Could you check a few things on this drawing? It's one solid part, dimensions in mm from its lowest x, y, z. A direction names the side the tool comes from. Give positions to 0.01 mm unless a question says otherwise; leave off trailing zeros. Write each loop counter-clockwise with the first axis right and the second up, starting at its lowest first coordinate (ties: lowest second). Pieces come first, ordered by that corner, then holes. Notation, with made-up numbers: M -6,-2 L 13,-2 A21 cw 13,7 Z; hole C 62.25,71.5 d3. An arc over 180 degrees is marked long. Use CSV: the item, a comma, the result in double quotes. Start each with the question number.
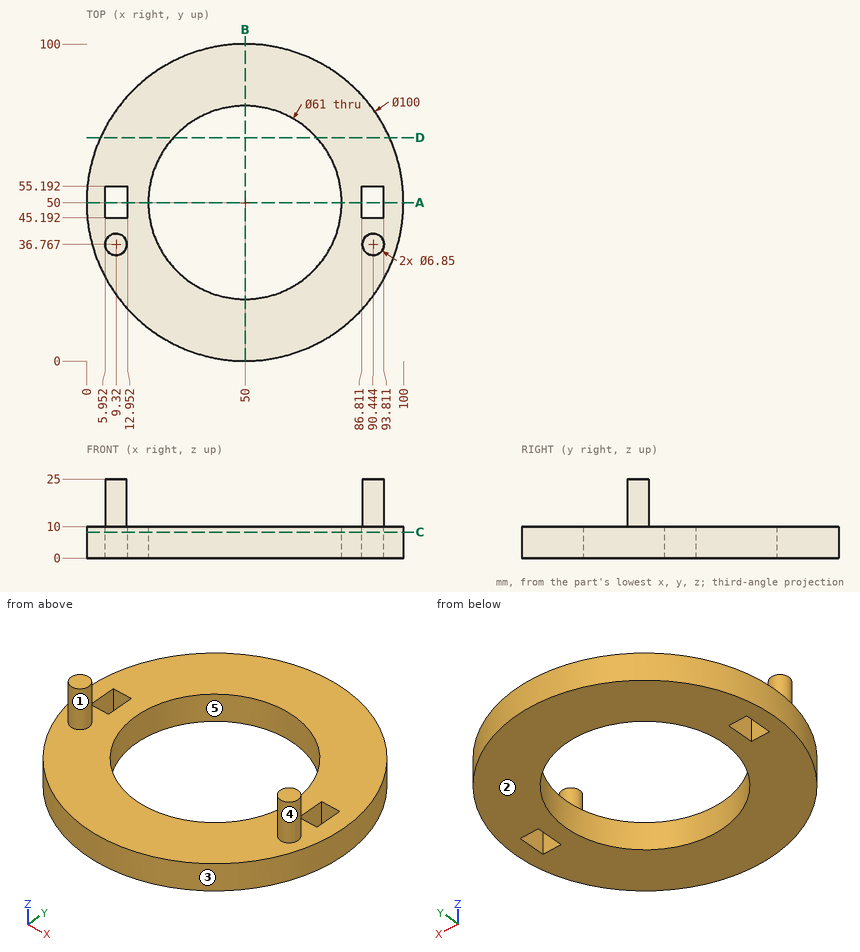
(1) Please list where these lines run through material, in increasing order: L1, parallel to Y at x = 50, z = 2.5; L2, parallel to Z at x = 10.5, y = 64; L3, parallel to Y at x = 88, z = 4.5 (1 decimal). Write a range as [from, to].
(2) I want a section at B-B (x = 50). Write out the boundary of the cut face in (y, z), and give its area (3 significant figures).
(3) Will these pins go through, and if not, where does the flat tip stop? pin 1 Ø10 at (y, z) = (13, 11.5) entering from -X (1 decimal); pin 2 Ø1 at (x, z) = (45.5, 8) entering from -Y; pin 3 Ø7.5 at (x, z) = (8, 4.5) entering from -Y; pin 4 Ø11 at (y, z) = (50.5, 3.5) entering from -X.
(4) Which directions (+Z, -Z, +X, -X, +Y, -Y) give clear straight access to the entire face, cutting with the end or side of a thin tool? Please do the marked faces 4 and 5.
(5) I want a section at C-C (z = 8.25). Write out the boundary of the cut face in (x, y), and give its area (3 significant figures).
(6) Thinking about a two-plate mould opening in X: for the marked faces 1, 2 and 3, which applies, released by +X, released by -X, zero draft, split by the parting line, or undercut?
(7) I want a section at D-D (y = 70.5). Write out the boundary of the cut face in (x, z) (1 decimal).
(8) I want a section at A-A (y = 50). Write out the boundary of the cut face in (x, z), and give its area (3 significant figures).
Geometry results:
1,L1,"y = [0, 19.5], [80.5, 100]"
1,L2,"z = [0, 10]"
1,L3,"y = [17.5, 45.2], [55.2, 82.5]"
2,outline,"M 0,0 L 19.5,0 L 19.5,10 L 0,10 Z; M 80.5,0 L 100,0 L 100,10 L 80.5,10 Z"
2,area,"390 mm2"
3,pin 1,"stops at x = 11.8"
3,pin 2,"stops at y = 0.16"
3,pin 3,"stops at y = 17.8"
3,pin 4,"stops at x = 0"
4,face 4,"+Z"
4,face 5,"+Z, -Z"
5,outline,"C 50,50 d100; hole M 5.95,45.19 L 12.95,45.19 L 12.95,55.19 L 5.95,55.19 Z; hole C 50,50 d61; hole M 86.81,45.19 L 93.81,45.19 L 93.81,55.19 L 86.81,55.19 Z"
5,area,"4,790 mm2"
6,face 1,"undercut"
6,face 2,"zero draft"
6,face 3,"split by the parting line"
7,outline,"M 4.4,0 L 27.4,0 L 27.4,10 L 4.4,10 Z; M 72.6,0 L 95.6,0 L 95.6,10 L 72.6,10 Z"
8,outline,"M 0,0 L 5.95,0 L 5.95,10 L 0,10 Z; M 12.95,0 L 19.5,0 L 19.5,10 L 12.95,10 Z; M 80.5,0 L 86.81,0 L 86.81,10 L 80.5,10 Z; M 93.81,0 L 100,0 L 100,10 L 93.81,10 Z"
8,area,"250 mm2"
